from build123d import *

# Parameters (mm, degrees)
SKETCH1_R               = 5.75
CYLINDERBASE_DEPTH      = 30.07
SKETCH2_R               = 3.34
THROUGHHOLE_DEPTH       = 31.07
BOSS_EXTRUDE2_DEPTH     = 6.2
SKETCH4_R               = 2
CUT_EXTRUDE2_DEPTH      = 31.07
SKETCH5_R               = 1.625
CUT_EXTRUDE3_DEPTH      = 7.235382907
CUT_EXTRUDE3_DEPTH_BACK = 7.235382907


with BuildPart() as part:
    # Sketch1 → cylinderBase (new body)
    with BuildSketch(Plane(origin=(0, 0, 0), x_dir=(1, 0, 0), z_dir=(0, 1, 0))):
        Circle(SKETCH1_R)
    extrude(amount=CYLINDERBASE_DEPTH)

    # Sketch2 → throughHole (cut, through all)
    with BuildSketch(Plane(origin=(0, 30.07, 0), x_dir=(1, 0, 0), z_dir=(0, 1, 0))):
        Circle(SKETCH2_R)
    extrude(amount=-THROUGHHOLE_DEPTH, mode=Mode.SUBTRACT)

    # Sketch3 → Boss-Extrude2 (add)
    with BuildSketch(Plane(origin=(0, 30.07, 0), x_dir=(1, 0, 0), z_dir=(0, 1, 0))):
        Polygon((0, -7.2), (6.235382907, -3.6), (6.235382907, 3.6), (0, 7.2), (-6.235382907, 3.6), (-6.235382907, -3.6), align=None)
    extrude(amount=-BOSS_EXTRUDE2_DEPTH)

    # Sketch4 → Cut-Extrude2 (cut, through all)
    with BuildSketch(Plane(origin=(0, 30.07, 0), x_dir=(1, 0, 0), z_dir=(0, 1, 0))):
        Circle(SKETCH4_R)
    extrude(amount=-CUT_EXTRUDE2_DEPTH, mode=Mode.SUBTRACT)

    # Sketch5 → Cut-Extrude3 (cut, two sides)
    with BuildSketch(Plane(origin=(0, 0, 0), x_dir=(0, 0, -1), z_dir=(1, 0, 0))) as cut_extrude3_sk:
        with Locations((0, 5.475)):
            Circle(SKETCH5_R)
    extrude(amount=CUT_EXTRUDE3_DEPTH, mode=Mode.SUBTRACT)
    extrude(cut_extrude3_sk.sketch, amount=-CUT_EXTRUDE3_DEPTH_BACK, mode=Mode.SUBTRACT)


solid = part.part
Geometry check sheet. Reference: the model listing, model coordinates, mm. A direction names the side the tool comes from. Round coordinates to 2 decimals unless told otherwise and drop trailing zeros. Write each loop counter-clockwise with the first axis right and the second up, starting at its lowest first coordinate (ties: lowest second). Pieces come first, ordered by that corner, then holes. Notation, with made-up numbers: (81.25, 6) - (112.25, 6) arc R32 cw to (112.25, 38) - close; hole circle Ø9 at (67.5, 82). An arc over 180 degrees is marked (long way). One line per item, written item: value.
1. Scan lines: L1, parallel to Y at x = -4.7, z = 0; L2, parallel to X at y = 27, z = 0; L3, parallel to Z at x = 0, y = 18. Record each from-to range of solid material in increasing order.
The answers:
L1: y = 0 to 3.85, 7.1 to 30.07
L2: x = -6.24 to -2, 2 to 6.24
L3: z = -5.75 to -3.34, 3.34 to 5.75
2. Cross-section at D-D on z = 5. Record the boundary of the cut face in (x, y), and give its area (3 significant figures).
The answers:
outline: (-3.81, 23.87) - (-2.84, 23.87) - (-2.84, 0) - (2.84, 0) - (2.84, 23.87) - (3.81, 23.87) - (3.81, 30.07) - (-3.81, 30.07) - close
area: 183 mm^2
3. Set-up check for faces 1 (the face through (0, 23.87, 6)), 2 (the face through (3.161, 27.013, -5.375)): record each of +Z, -Z, +X, -X, +Y, -Y from which the full face is reachable in a straight line by a thin tool's end or side.
The answers:
face 1: -Y
face 2: -Z, +X, +Y, -Y
4. Mould release check, pull along X, two halves, no side actions. Record for faces 3 (the face through (3.085, 12.102, 1.279)), 4 (the face through (5.484, 11.768, -1.727)), 5 (the face through (-3.074, 27.013, -5.425)): released by +X, released by -X, zero draft, split by the parting line, or undercut.
The answers:
face 3: undercut
face 4: split by the parting line
face 5: released by -X
5. Depth check by flat-ended pin: pin 1 Ø2 at (x, y) = (0.5, 4.5) entering from +Z; pin 2 Ø5 at (x, y) = (3, 15) entering from -Z; pin 3 Ø2 at (x, z) = (1.5, 1.5) entering from -Y. Enter the tip coordinate at first touch or a pass-through.
The answers:
pin 1: stops at z = 5.75
pin 2: stops at z = -5.73
pin 3: stops at y = 23.87
6. Cross-section at B-B on x = 4.75. Record the boundary of the cut face in (y, z) (3 decimals).
The answers:
outline: (0, -3.24) - (23.87, -3.24) - (23.87, -4.458) - (30.07, -4.458) - (30.07, 4.458) - (23.87, 4.458) - (23.87, 3.24) - (0, 3.24) - close; hole circle Ø3.25 at (5.475, 0)
7. Cross-section at A-A on z = 0. Record the boundary of the cut face in (x, y), and give its area (3 significant figures).
The answers:
outline: (-6.24, 23.87) - (-5.75, 23.87) - (-5.75, 7.1) - (-3.34, 7.1) - (-3.34, 23.87) - (-2, 23.87) - (-2, 30.07) - (-6.24, 30.07) - close; (-5.75, 0) - (-3.34, 0) - (-3.34, 3.85) - (-5.75, 3.85) - close; (2, 23.87) - (3.34, 23.87) - (3.34, 7.1) - (5.75, 7.1) - (5.75, 23.87) - (6.24, 23.87) - (6.24, 30.07) - (2, 30.07) - close; (3.34, 0) - (5.75, 0) - (5.75, 3.85) - (3.34, 3.85) - close
area: 152 mm^2
8. Cross-section at C-C on y = 12.5. Record the boundary of the cut face in (x, z).
The answers:
outline: circle Ø11.5 at (0, 0); hole circle Ø6.68 at (0, 0)
